from build123d import *

# Parameters (mm, degrees)
BOSS_EXTRUDE1_DEPTH = 14.224
SKETCH2_R           = 1.524
CUT_EXTRUDE1_DEPTH  = 48.306775498
SKETCH3_R           = 1.905
CUT_EXTRUDE2_DEPTH  = 38.388604586


with BuildPart() as part:
    # Sketch1 → Boss-Extrude1 (new body)
    with BuildSketch(Plane(origin=(0, 0, 0), x_dir=(0, 0, -1), z_dir=(1, 0, 0))):
        with BuildLine():
            Line((-17.230995516, 26.416), (-17.230995516, 12.7))
            ThreePointArc((-17.230995516, 12.7), (-13.511251637, 3.719743879), (-4.530995516, 0))
            Line((-4.530995516, 0), (14.265004484, 0))
            Line((14.265004484, 0), (14.265004484, -5.08))
            Line((14.265004484, -5.08), (-17.230995516, -5.08))
            Line((-17.230995516, -5.08), (-22.310995516, -5.08))
            Line((-22.310995516, -5.08), (-22.310995516, 26.416))
            Line((-22.310995516, 26.416), (-17.230995516, 26.416))
        make_face()
    extrude(amount=BOSS_EXTRUDE1_DEPTH)

    # Sketch2 → Cut-Extrude1 (cut, through all)
    with BuildSketch(Plane.XY.offset(22.310995516)):
        with Locations((7.112, 19.558)):
            Circle(SKETCH2_R)
    extrude(amount=-CUT_EXTRUDE1_DEPTH, mode=Mode.SUBTRACT)

    # Sketch3 → Cut-Extrude2 (cut, through all)
    with BuildSketch(Plane(origin=(0, 0, 0), x_dir=(1, 0, 0), z_dir=(0, 1, 0))):
        with Locations(Location((7.112, 8.49810052, 0), (0, 0, 270))):
            Circle(SKETCH3_R)
    extrude(amount=-CUT_EXTRUDE2_DEPTH, mode=Mode.SUBTRACT)


solid = part.part
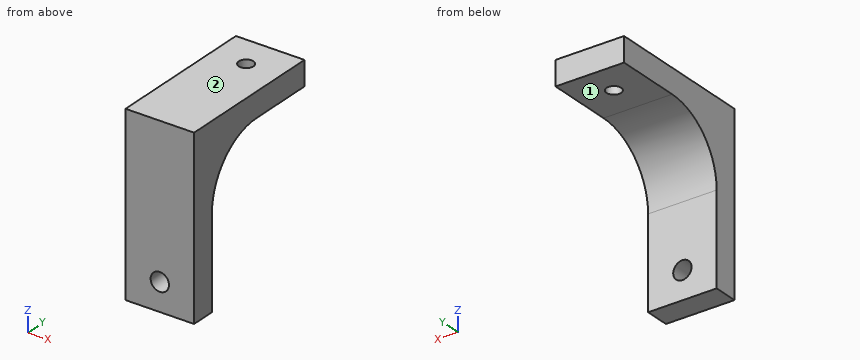
For this review, take the finished solid that the model builds, in its own axes (mm). Face numbers are marked on the shaded views. A direction names the side the tool comes from. Coordinates: 2 decimals unless noted, no trailing zeros. Loops run counter-clockwise (first coordinate to the right, second up) from the corner with the lowest first, then second, coordinate; pieces in that order, holes last. Notation, with made-up numbers: (-35, -23.75) - (-1, -23.75) arc R8 cw to (-1, -15.75) - close; hole circle Ø3 at (-0.5, -24.75). An arc over 180 degrees is marked (long way). Return JSON: item names as keys, results as strings.
Item 1: Take a section at A-A (x = 3). Give the boundary of the cut face in (y, z) (3 decimals).
Determined:
{"outline": "(-5.08, -14.265) - (0, -14.265) - (0, 4.531) arc R12.7 cw to (12.7, 17.231) - (26.416, 17.231) - (26.416, 22.311) - (-5.08, 22.311) - close"}
Item 2: Take a section at B-B (z = -8). Give the boundary of the cut face in (x, y), then the cut area to 3 significant figures.
Determined:
{"outline": "(0, -5.08) - (5.27, -5.08) - (5.27, 0) - (0, 0) - close; (8.95, -5.08) - (14.22, -5.08) - (14.22, 0) - (8.95, 0) - close", "area": "53.6 mm2"}
Item 3: Take a section at D-D (y = -1). Give the boundary of the cut face in (x, z) (3 decimals), then the cut area to 3 significant figures.
Determined:
{"outline": "(0, -14.265) - (14.224, -14.265) - (14.224, 22.311) - (0, 22.311) - close; hole circle Ø3.81 at (7.112, -8.498)", "area": "509 mm2"}
Item 4: Insertion check: pin 1 (10 mm diameter, centred on y = 7.5, z = 2.5, fed in from +X); pin 2 (5 mm diameter, centred on x = 7.112, y = 19.558, fed in from -Z); pin 3 (4.5 mm diameter, centred on x = 9.5, z = -7.5, fed in from +Y). Each pin has a flat end and moves straight along its axis. Give the tip position at first contact, or say it passes through.
Determined:
{"pin 1": "passes through", "pin 2": "stops at z = 17.23", "pin 3": "stops at y = 0"}
Item 5: For the marked faces 1 and 2, list the 3-axis set-ups (+Z, -Z, +X, -X, +Y, -Y) from which the entire face can be reached by the end or side of a thin tool; tool diameter is ignored.
Determined:
{"face 1": "-Z, +X, -X, +Y", "face 2": "+Z, +X, -X, +Y, -Y"}
Item 6: Take a section at C-C (x = 6.25). Give the boundary of the cut face in (y, z) (3 decimals).
Determined:
{"outline": "(-5.08, -14.265) - (0, -14.265) - (0, -10.197) - (-5.08, -10.197) - close; (-5.08, -6.799) - (0, -6.799) - (0, 4.531) arc R12.7 cw to (12.7, 17.231) - (18.301, 17.231) - (18.301, 22.311) - (-5.08, 22.311) - close; (20.815, 17.231) - (26.416, 17.231) - (26.416, 22.311) - (20.815, 22.311) - close"}
Item 7: For line 1 (Y direction, x = 3.75, z = -1); line 2 (Z direction, x = 3, y = 14.5); line 3 (X direction, y = 20.5, z = 20), list the stretches that pass through material, from the lowest coordinate up.
Determined:
{"line 1": "y = -5.08 to 0", "line 2": "z = 17.23 to 22.31", "line 3": "x = 0 to 5.91, 8.31 to 14.22"}
